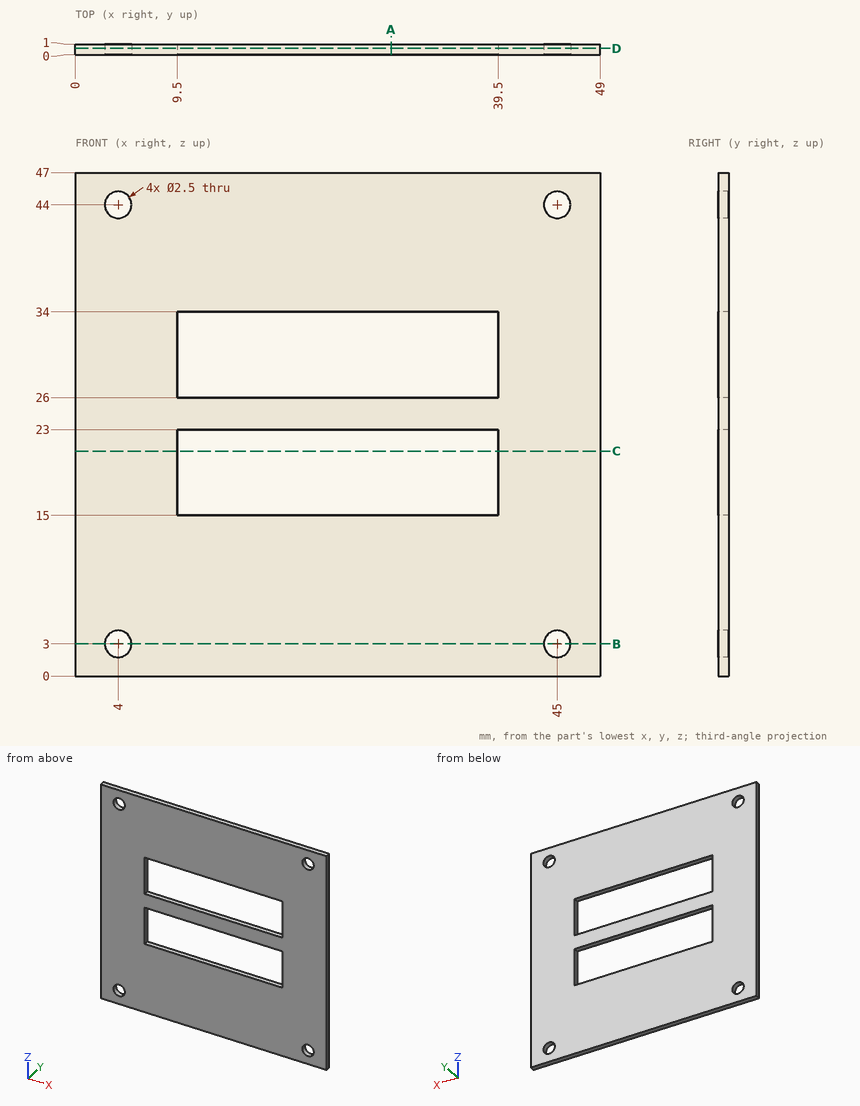
Could you check a few things on this drawing? It's one solid part, dimensions in mm from its lowest x, y, z. Give positions to 0.01 mm unless a question says otherwise; leave off trailing zeros. Write each loop counter-clockwise with the first axis right and the second up, starting at its lowest first coordinate (ties: lowest second). Pieces come first, ordered by that corner, then holes. Notation, with made-up numbers: (30, 37) -> (73, 37) arc R15 cw to (73, 46) -> close; hole circle Ø11 at (3.5, 74.25). An arc over 180 degrees is marked (long way). Answer as CSV lines item,"result". Start each with the question number.
(1) If we section it at D-D, the plane y = 0.6: Write out the boundary of the cut face in (x, z).
(2) If we section it at B-B, the plane z = 3: Write out the boundary of the cut face in (x, y).
(3) Please list where these lines run through material, in increasing order: line 1 (Z direction, x = 39, y = 0.9); line 2 (X direction, y = 0.5, z = 44); line 3 (X direction, y = 0.45, z = 22).
(4) If we section it at A-A, the plane x = 29.5: Write out the boundary of the cut face in (y, z), and give its area (3 significant figures).
(5) If we section it at C-C, the plane z = 21: Write out the boundary of the cut face in (x, y).
Answer list:
1,outline,"(0, 0) -> (49, 0) -> (49, 47) -> (0, 47) -> close; hole circle Ø2.5 at (4, 3); hole circle Ø2.5 at (4, 44); hole (9.5, 15) -> (39.5, 15) -> (39.5, 23) -> (9.5, 23) -> close; hole (9.5, 26) -> (39.5, 26) -> (39.5, 34) -> (9.5, 34) -> close; hole circle Ø2.5 at (45, 3); hole circle Ø2.5 at (45, 44)"
2,outline,"(0, 0) -> (2.75, 0) -> (2.75, 1) -> (0, 1) -> close; (5.25, 0) -> (43.75, 0) -> (43.75, 1) -> (5.25, 1) -> close; (46.25, 0) -> (49, 0) -> (49, 1) -> (46.25, 1) -> close"
3,line 1,"0 to 15, 23 to 26, 34 to 47"
3,line 2,"0 to 2.75, 5.25 to 43.75, 46.25 to 49"
3,line 3,"0 to 9.5, 39.5 to 49"
4,outline,"(0, 0) -> (1, 0) -> (1, 15) -> (0, 15) -> close; (0, 23) -> (1, 23) -> (1, 26) -> (0, 26) -> close; (0, 34) -> (1, 34) -> (1, 47) -> (0, 47) -> close"
4,area,"31.0 mm^2"
5,outline,"(0, 0) -> (9.5, 0) -> (9.5, 1) -> (0, 1) -> close; (39.5, 0) -> (49, 0) -> (49, 1) -> (39.5, 1) -> close"
